```python
from build123d import *

# Parameters (mm, degrees)
CHAMFER1_SIZE         = 1
TROU_TARAUD_M81_D     = 6.8
TROU_TARAUD_M81_DEPTH = 22
TROU_TARAUD_M81_TIP   = 2.042926105


with BuildPart() as part:
    # Sketch1 → Revolve1 (revolve)
    with BuildSketch(Plane.XY):
        Polygon((0, 70), (0, -78), (-6, -78), (-6, -10), (-17.5, -10), (-17.5, 0), (-6, 0), (-6, 70), align=None)
    revolve(axis=Axis((0, 34.427667765, 0), (0, -1, 0)))

    # Chamfer1
    chamfer1_edges = [part.edges().sort_by_distance(p)[0] for p in [
        (6, 70, 0),
        (17.5, 0, 0),
        (17.5, -10, 0),
        (6, -78, 0),
    ]]
    chamfer(chamfer1_edges, length=CHAMFER1_SIZE)

    # Trou taraudé M81
    with Locations(Plane(origin=(0, 70, 0), x_dir=(1, 0, 0), z_dir=(0, 1, 0))):
        with Locations((0, 0)):
            Hole(TROU_TARAUD_M81_D / 2, depth=TROU_TARAUD_M81_DEPTH)
            with Locations((0, 0, -(TROU_TARAUD_M81_DEPTH + TROU_TARAUD_M81_TIP / 2))):  # 118° drill point
                Cone(0, TROU_TARAUD_M81_D / 2, TROU_TARAUD_M81_TIP, mode=Mode.SUBTRACT)


solid = part.part
```
Here's how the part is built. I have some questions about the finished solid (model axes, mm). A direction names the side the tool comes from. Give positions to 0.01 mm unless a question says otherwise; leave off trailing zeros. Order: outer loops, then holes, each group sorted by start corner. A loop starts at its lowest first (then second) coordinate and runs counter-clockwise, first axis right, second up. Notation, with made-up numbers: (72, 69) - (80, 69) arc R20 cw to (80, 87) - close; hole circle Ø2 at (56.25, -12.5). An arc over 180 degrees is marked (long way). Answer as a JSON object with one key per item and string values. Group by question number.
Item 1: Please list where these lines run through material, in increasing order: probe 1 along Z at (x, y) = (0, 63.75); probe 2 along Y at (x, z) = (16, -2.5); probe 3 along Z at (x, y) = (0.5, 32).
Item 2: If we section it at B-B on y = 1.5: Please give me the cut outline in (x, z).
Item 3: For P1, Ø10, axis at y = 55, z = 0.5, coming from the -X side; P2, Ø12, axis at x = -12, y = -3.5, coming from the +Z side; P3, Ø2, axis at y = 40, z = -6, coming from the +X side, each with a flat end and sliding along its axis, tell me the tip position at first contact or that it passes through.
Item 4: Which directions (+Z, -Z, +X, -X, +Y, -Y) give clear straight access to the entire face, cutting with the end or side of a thin tool? Please do faces 1 (the flat face through (0, -78, 0)), 2 (the flat face through (0, 0, 7)).
Item 5: If we section it at A-A on y = 51.5: Please give me the cut outline in (x, z).
Item 6: If we mould it in two halves opening along Z, with no side actions, what happens to faces 3 (the conical face through (-0.128, 46.312, 0.576)), 4 (the cylindrical face through (6, -43, 0)), 5 (the flat face through (0, -10, 7))? For each: pulls with the +Z half, pulls with the -Z half, needs draft (parallel to the pull), parting line crosses it, or undercut.
Result set:
{
 "1": {"probe 1": "-6 to -3.4, 3.4 to 6", "probe 2": "-10 to 0", "probe 3": "-5.98 to 5.98"},
 "2": {"outline": "circle Ø12 at (0, 0)"},
 "3": {"P1": "x = -6", "P2": "z = 16.44", "P3": "x = 3.32"},
 "4": {"face 1": "+Z, -Z, +X, -X, -Y", "face 2": "+Y"},
 "5": {"outline": "circle Ø12 at (0, 0); hole circle Ø6.8 at (0, 0)"},
 "6": {"face 3": "undercut", "face 4": "parting line crosses it", "face 5": "needs draft"}
}
